Part model, mm, in its own coordinate system. A direction names the side the tool comes from. Round coordinates to 2 decimals unless told otherwise and drop trailing zeros. Write each loop counter-clockwise with the first axis right and the second up, starting at its lowest first coordinate (ties: lowest second). Pieces come first, ordered by that corner, then holes. Notation, with made-up numbers: M -2,76.5 L 21,76.5 A20 cw 21,115.5 Z; hole C -23.75,-20.75 d8. An arc over 180 degrees is marked long. Answer as a JSON object with one key per item and string values. Group by question number.
1. Which spindle directions (+Z, -Z, +X, -X, +Y, -Y) get a long thin tool onto all of the face, cutting with end or side? Do faces 1 (the face through (-1, 1.2, 3)), 2 (the face through (20, 1.2, 3)), 3 (the face through (18.82, -6, 4)). Say none if no direction does.
2. Band-saw the part on C-C, the plane z = 0.5. Write the cut outline in (x, y).
3. Band-saw the part on B-B, the plane z = 4.25. Write the cut outline in (x, y).
4. Band-saw the part on A-A, the plane x = -2. Write the cut outline in (y, z) (3 decimals), plus the area to 3 significant figures.
5. Two-plate mould, pull along Z, no slides. Class faces 4 (the face through (19.99, 0.61, 3.46)), 5 (the face through (1.66, 5.08, 5.59)), 6 (the face through (0, -6, 4)): +Z half, -Z half, draft (parallel to the pull), parting line (faces both ways), or undercut.
6. Drill centre lines: line 1 (Z direction, x = -2, y = 0.4) (3 decimals); line 2 (Y direction, x = 6.5, z = 5.5); line 3 (X direction, y = 2.5, z = 4.25). Where is each one in solid material? Low to high. Write a range as from..to.
7. Band-saw the part on D-D, the plane x = 1.75. Write the cut outline in (y, z).
8. Drop flat-ended pins along their axis: pin 1 (1.9 mm diameter, centred on x = 21.5, z = 5.5, fed in from +Y); pin 2 (3 mm diameter, centred on y = 4, z = 4, fed in from +X); pin 3 (1.9 mm diameter, centred on x = 21, z = 5.5, fed in from -Y); pin 4 (1.4 mm diameter, centred on x = -2, z = 3.805, fed in from -Y) (3 decimals). Give the stop position or say it passes through.
from build123d import *

# Parameters (mm, degrees)
BOSS_EXTRUDE1_DEPTH = 7.61
SKETCH2_R           = 0.9
CUT_EXTRUDE1_DEPTH  = 1.2
SKETCH3_R           = 2.926040877
BOSS_EXTRUDE2_DEPTH = 1.49
SKETCH4_R           = 1.393854302
BOSS_EXTRUDE3_DEPTH = 2.7


with BuildPart() as part:
    # Sketch1 → Boss-Extrude1 (new body)
    with BuildSketch(Plane.XY):
        Polygon((0, 0), (0, -11.32), (18.82, -11.32), (18.82, 0), (22.7, 0), (22.7, 1.2), (18.82, 1.2), (18.82, 4.35), (0, 4.35), (0, 1.2), (-3.88, 1.2), (-3.88, 0), align=None)
    extrude(amount=BOSS_EXTRUDE1_DEPTH)

    # Sketch2 → Cut-Extrude1 (cut)
    with BuildSketch(Plane(origin=(0, 1.2, 0), x_dir=(1, 0, 0), z_dir=(0, 1, 0))):
        with Locations(Location((20.82, -3.805, 0), (0, 0, 180))):
            Circle(SKETCH2_R)
        with Locations(Location((-2, -3.805, 0), (0, 0, 180))):
            Circle(SKETCH2_R)
    extrude(amount=-CUT_EXTRUDE1_DEPTH, mode=Mode.SUBTRACT)

    # Sketch3 → Boss-Extrude2 (add)
    with BuildSketch(Plane(origin=(0, 4.35, 0), x_dir=(1, 0, 0), z_dir=(0, 1, 0))):
        with Locations((3.977412239, -3.805)):
            Circle(SKETCH3_R)
    extrude(amount=BOSS_EXTRUDE2_DEPTH)

    # Sketch4 → Boss-Extrude3 (add)
    with BuildSketch(Plane(origin=(0, 5.84, 0), x_dir=(1, 0, 0), z_dir=(0, 1, 0))):
        with Locations((3.977412239, -3.805)):
            Circle(SKETCH4_R)
    extrude(amount=BOSS_EXTRUDE3_DEPTH)


solid = part.part
Worked answers:
{
 "1": {"face 1": "+Z, -Z, -X, +Y", "face 2": "+Z, -Z, +X, +Y", "face 3": "+Z, -Z, +X, -Y"},
 "2": {"outline": "M -3.88,0 L 0,0 L 0,-11.32 L 18.82,-11.32 L 18.82,0 L 22.7,0 L 22.7,1.2 L 18.82,1.2 L 18.82,4.35 L 0,4.35 L 0,1.2 L -3.88,1.2 Z"},
 "3": {"outline": "M -3.88,0 L -2.78,0 L -2.78,1.2 L -3.88,1.2 Z; M -1.22,0 L 0,0 L 0,-11.32 L 18.82,-11.32 L 18.82,0 L 20.04,0 L 20.04,1.2 L 18.82,1.2 L 18.82,4.35 L 6.87,4.35 L 6.87,5.84 L 5.3,5.84 L 5.3,8.54 L 2.66,8.54 L 2.66,5.84 L 1.09,5.84 L 1.09,4.35 L 0,4.35 L 0,1.2 L -1.22,1.2 Z; M 21.6,0 L 22.7,0 L 22.7,1.2 L 21.6,1.2 Z"},
 "4": {"outline": "M 0,0 L 1.2,0 L 1.2,2.905 L 0,2.905 Z; M 0,4.705 L 1.2,4.705 L 1.2,7.61 L 0,7.61 Z", "area": "6.97 mm^2"},
 "5": {"face 4": "undercut", "face 5": "parting line", "face 6": "draft"},
 "6": {"line 1": "z = 0..2.905, 4.705..7.61", "line 2": "y = -11.32..4.35", "line 3": "x = 0..18.82"},
 "7": {"outline": "M -11.32,0 L 4.35,0 L 4.35,1.91 L 5.84,1.91 L 5.84,5.7 L 4.35,5.7 L 4.35,7.61 L -11.32,7.61 Z"},
 "8": {"pin 1": "stops at y = 1.2", "pin 2": "stops at x = 18.82", "pin 3": "stops at y = 0", "pin 4": "passes through"}
}
